```python
from build123d import *


with BuildPart() as part:
    # Sweep1: sweep along a path in Sketch4
    with BuildLine(Plane.XY) as sweep1_path:
        Line((0, -65.154874543), (0, 56.003125457))
        ThreePointArc((0, 56.003125457), (0.185987194, 56.452138263), (0.635, 56.638125457))
        Line((0.635, 56.638125457), (121.793, 56.638125457))
        ThreePointArc((121.793, 56.638125457), (122.242012806, 56.452138263), (122.428, 56.003125457))
        Line((122.428, 56.003125457), (122.428, -65.154874543))
        ThreePointArc((122.428, -65.154874543), (122.242012806, -65.603887349), (121.793, -65.789874543))
        Line((121.793, -65.789874543), (0.635, -65.789874543))
        ThreePointArc((0.635, -65.789874543), (0.185987194, -65.603887349), (0, -65.154874543))
    # Sketch3 → Sweep1 (sweep)
    with BuildSketch(Plane(origin=(0, 0, 0), x_dir=(1, 0, 0), z_dir=(0, 1, 0))):
        with BuildLine():
            Line((0, 0), (0, 10.72500014))
            Line((0, 10.72500014), (-25.4, 10.72500014))
            Line((-25.4, 10.72500014), (-25.4, 5.64500014))
            Line((-25.4, 5.64500014), (-6.535, 5.64500014))
            ThreePointArc((-6.535, 5.64500014), (-6.085987194, 5.459012946), (-5.9, 5.01000014))
            Line((-5.9, 5.01000014), (-5.9, -13.21999986))
            ThreePointArc((-5.9, -13.21999986), (-6.085987194, -13.669012666), (-6.535, -13.85499986))
            Line((-6.535, -13.85499986), (-25.4, -13.85499986))
            Line((-25.4, -13.85499986), (-25.4, -18.93499986))
            Line((-25.4, -18.93499986), (0, -18.93499986))
            Line((0, -18.93499986), (0, 0))
        make_face()
    sweep(path=sweep1_path.line)


solid = part.part
```
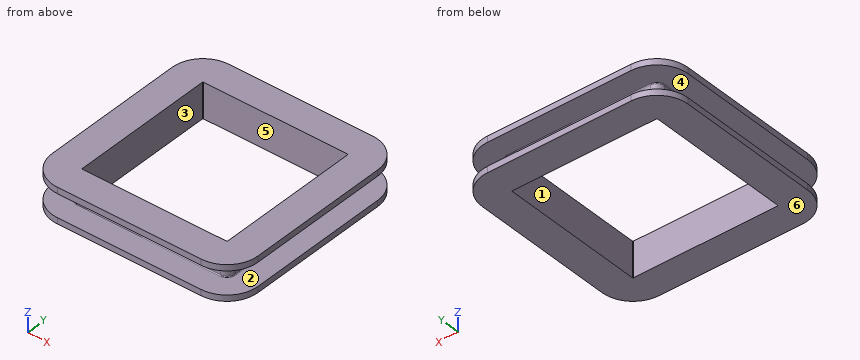
Here's how the part is built. I have some questions about the finished solid (model axes, mm). Face numbers are marked on the shaded views. A direction names the side the tool comes from. Coordinates: 2 decimals unless noted, no trailing zeros. Write each loop counter-clockwise with the first axis right and the second up, starting at its lowest first coordinate (ties: lowest second). Pieces come first, ordered by that corner, then holes. Notation, with made-up numbers: (63, 25.25) - (117, 25.25) arc R21 ccw to (117, 45.25) - close; hole circle Ø9 at (72, -24). An arc over 180 degrees is marked (long way). One line per item, written item: value.
1) I need wall thicknesses on line 1 along Z through (x, y) = (129, 56) (3 decimals); line 2 along Y through (x, z) = (121.5, 9.5); line 3 along X through (y, z) = (-34.5, -7). Which ranges of each line are inside material? Lowest first, please.
Model answer:
line 1: z = -10.725 to -5.645, 13.855 to 18.935
line 2: y = -71.69 to -65.79, 56.64 to 62.54
line 3: x = -25.4 to 0, 122.43 to 147.83
2) On a 3-axis mill with a long thin cutter (end or side, diameter ignored), from which of +Z, -Z, +X, -X, +Y, -Y can I reach the whole of each face in a straight line? I mean the marked faces 4, 5 and 6. Say none if no direction works.
Model answer:
face 4: none
face 5: +Z, -Z
face 6: -Z, +X, -X, +Y, -Y
3) Suppose I cut it at D-D on x = 137. Write out the boundary of the cut face in (y, z) (3 decimals).
Model answer:
outline: (-86.287, -10.725) - (77.135, -10.725) - (77.135, -5.645) - (-86.287, -5.645) - close; (-86.287, 13.855) - (77.135, 13.855) - (77.135, 18.935) - (-86.287, 18.935) - close
4) Suppose I cut it at B-B on x = 37. Write out the boundary of the cut face in (y, z) (3 decimals), and give its area (3 significant figures).
Model answer:
outline: (-91.19, -10.725) - (-65.79, -10.725) - (-65.79, 18.935) - (-91.19, 18.935) - (-91.19, 13.855) - (-72.325, 13.855) arc R0.635 cw to (-71.69, 13.22) - (-71.69, -5.01) arc R0.635 cw to (-72.325, -5.645) - (-91.19, -5.645) - close; (56.638, -10.725) - (82.038, -10.725) - (82.038, -5.645) - (63.173, -5.645) arc R0.635 cw to (62.538, -5.01) - (62.538, 13.22) arc R0.635 cw to (63.173, 13.855) - (82.038, 13.855) - (82.038, 18.935) - (56.638, 18.935) - close
area: 747 mm²
5) We'd pull the mould along X, two halves only. Please class the marked faces 1, 2 and 3: pulls with the +X half, pulls with the -X half, needs draft (parallel to the pull), parting line crosses it, or undercut.
Model answer:
face 1: undercut
face 2: needs draft
face 3: undercut
6) Suppose I cut it at A-A on z = 6.25. Write out the boundary of the cut face in (x, y) (3 decimals).
Model answer:
outline: (-5.9, -65.155) arc R6.535 ccw to (0.635, -71.69) - (121.793, -71.69) arc R6.535 ccw to (128.328, -65.155) - (128.328, 56.003) arc R6.535 ccw to (121.793, 62.538) - (0.635, 62.538) arc R6.535 ccw to (-5.9, 56.003) - close; hole (0, -65.155) arc R0.635 ccw to (0.635, -65.79) - (121.793, -65.79) arc R0.635 ccw to (122.428, -65.155) - (122.428, 56.003) arc R0.635 ccw to (121.793, 56.638) - (0.635, 56.638) arc R0.635 ccw to (0, 56.003) - close
7) Suppose I cut it at C-C on y = 26. Write out the boundary of the cut face in (x, z) (3 decimals).
Model answer:
outline: (-25.4, -10.725) - (0, -10.725) - (0, 18.935) - (-25.4, 18.935) - (-25.4, 13.855) - (-6.535, 13.855) arc R0.635 cw to (-5.9, 13.22) - (-5.9, -5.01) arc R0.635 cw to (-6.535, -5.645) - (-25.4, -5.645) - close; (122.428, -10.725) - (147.828, -10.725) - (147.828, -5.645) - (128.963, -5.645) arc R0.635 cw to (128.328, -5.01) - (128.328, 13.22) arc R0.635 cw to (128.963, 13.855) - (147.828, 13.855) - (147.828, 18.935) - (122.428, 18.935) - close
8) I'm going to push flat-ended pins straight in: P1, Ø15, axis at y = 14, z = 2, coming from the -X side; P2, Ø9, axis at x = 42, z = 3.5, coming from the -Y side; P3, Ø1, axis at x = 95.5, z = 9.5, coming from the +Y side. Where does each tip first touch, or does it pass through?
Model answer:
P1: stops at x = -6.13
P2: stops at y = -71.69
P3: stops at y = 62.54
